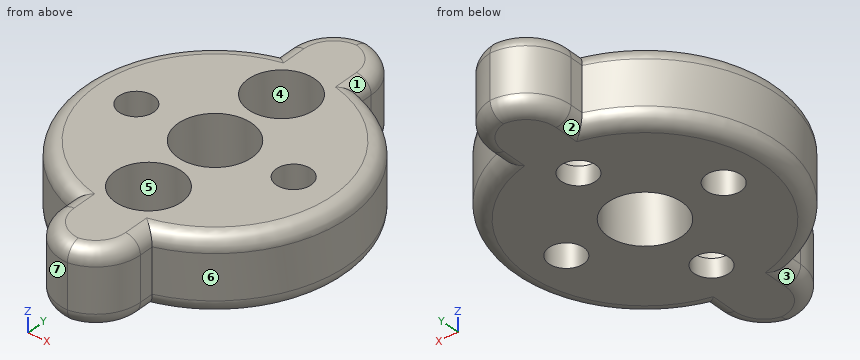
Autodesk Inventor part; units mm, degrees
ref_plane "YZ Plane" through (0, 0, 0) normal (1, 0, 0) x (0, 1, 0)
ref_plane "XZ Plane" through (0, 0, 0) normal (0, 1, 0) x (-1, 0, 0)
ref_plane "XY Plane" through (0, 0, 0) normal (0, 0, 1) x (1, 0, 0)
sketch "Sketch1" plane through (0, 0, 0) normal (0, 0, 1) x (1, 0, 0)
  circle A0 centre (0, 0) radius 11.43
  circle A1 centre (-6.75, 0) radius 1.5
  circle A2 centre (0, 0) radius 1.5
  circle A3 centre (6.75, 0) radius 1.5
  line L0 (0, 0) -> (0, 6.985)
  line L1 (0, 0) -> (0, -6.985)
  circle A4 centre (0, 6.985) radius 1.4986
  circle A5 centre (0, -6.985) radius 1.4986
  circle A6 centre (0, 0) radius 3.175
  arc A7 (0.31, -15.875) -> (3.5, -12.1158) centre (-0.31, -12.1158) ccw
  line L2 (3.5, -12.1158) -> (3.5, 12.1158)
  arc A8 (3.5, 12.1158) -> (0.31, 15.875) centre (-0.31, 12.1158) ccw
  arc A9 (0.31, 15.875) -> (-3.5, 12.065) centre (0.31, 12.065) ccw
  line L3 (-3.5, 12.065) -> (-3.5, -12.065)
  arc A10 (-3.5, -12.065) -> (0.31, -15.875) centre (0.31, -12.065) ccw
  circle A11 centre (0, 6.985) radius 1.5
  circle A12 centre (0, -6.985) radius 1.5
  line L4 (3.5, 0) -> (-3.5, 0)
  line L5 (0, 0) -> (0, 6.985)
  point P0 (3.5, -10.8809)
  point P1 (-3.5, -10.8809)
  point P2 (-3.5, 10.8809)
  point P3 (3.5, 10.8809)
  dimension "d0" = 22.86
  dimension "d1" = 6.985
  dimension "d2" = 6.985
  dimension "d3" = 2.9972
  dimension "d4" = 2.9972
  dimension "d7" = 6.35
extrude "Extrusion1" add sketch "Sketch1" along normal blind 6.35 contours A0 L2 | L2 L4 A6 L3 A0 | A0 L3 A9 A8 L2 | L2 A7 A10 L3 A0 | A0 L3 L4 A6 L2 | L3 A0
fillet "Fillet2" radius 1.27 20 edges at (11.43, 0, 0) (11.43, 0, 6.35) (-11.43, 0, 0) (-11.43, 0, 6.35) (3.5, 11.4984, 6.35) (2.595, 14.5809, 6.35) (-3.5, 11.473, 6.35) (-2.3841, 14.7591, 6.35) (-3.5, 11.473, 0) (-2.3841, 14.7591, 0) (3.5, 11.4984, 0) (2.595, 14.5809, 0) (2.595, -14.5809, 6.35) (3.5, -11.4984, 6.35) (-3.5, -11.473, 6.35) (-2.3841, -14.7591, 6.35) (3.5, -11.4984, 0) (2.595, -14.5809, 0) (-3.5, -11.473, 0) (-2.3841, -14.7591, 0)
sketch "Sketch3" plane through (0, 0, 6.35) normal (0, 0, 1) x (1, 0, 0)
  circle A0 centre (0, 6.985) radius 1.4986
  circle A1 centre (0, 6.985) radius 2.8575
  circle A2 centre (0, -6.985) radius 1.4986
  circle A3 centre (0, -6.985) radius 2.8575
  point P0 (0, 0)
  dimension "d12" = 5.715
  dimension "d13" = 5.715
extrude "Extrusion2" cut sketch "Sketch3" against normal blind 4.7625
properties part number "turning_cap"
The model under review builds one solid part; all positions refer to its coordinate system, in mm. Face numbers are marked on the shaded views. A direction names the side the tool comes from. Give positions to 0.01 mm unless a question says otherwise; leave off trailing zeros. Write each loop counter-clockwise with the first axis right and the second up, starting at its lowest first coordinate (ties: lowest second). Pieces come first, ordered by that corner, then holes. Notation, with made-up numbers: (-19.5, 32.25) -> (-0.5, 32.25) arc R23 ccw to (-0.5, 41.25) -> close; hole circle Ø8 at (73, 49.25). An arc over 180 degrees is marked (long way). Answer in a Markdown table with one row per item.
1) Mouldability with a two-part tool opening along Y and no side actions: class the marked faces 5, 6 and 7 as +Y half, -Y half, draft (parallel to the pull), parting line (faces both ways), or undercut.
Worked answers:
| item | result |
|---|---|
| face 5 | undercut |
| face 6 | parting line |
| face 7 | -Y half |
2) For L1, parallel to Y at x = -7.5, z = 5; L2, parallel to Z at x = 1.5, y = 14; L3, parallel to Y at x = 1, z = 6, list the stretches that pass through material, from the lowest coordinate up. Write a range as [from, to].
Worked answers:
| item | result |
|---|---|
| L1 | [-8.63, -1.3], [1.3, 8.63] |
| L2 | [0, 6.35] |
| L3 | [-15.27, -9.66], [-4.31, -3.01], [3.01, 4.31], [9.66, 15.27] |
3) Clearance check with flat-ended pins moving along their axes: P1, Ø3.5, axis at x = 0, y = -6.985, coming from the +Z side; P2, Ø4, axis at x = -5, y = -12, coming from the -Z side; P3, Ø0.9, axis at y = -11.5, z = 3, coming from the -X side; P4, Ø1.8, axis at x = 0, y = -6.985, coming from the -Z side. State where each tip first meets the part, or that it passes through.
Worked answers:
| item | result |
|---|---|
| P1 | z = 1.59 |
| P2 | z = 0.26 |
| P3 | x = -3.5 |
| P4 | through |
4) Tool access review of the marked faces 1, 2, 3 and 4: name each direction out of +Z, -Z, +X, -X, +Y, -Y from which nothing blocks a thin tool from reaching the whole face with its end or side.
Worked answers:
| item | result |
|---|---|
| face 1 | +Z, +X, +Y |
| face 2 | -Z, -X, +Y |
| face 3 | -Z, -X, -Y |
| face 4 | +Z |
5) Add section A-A on y = 0. State the section outline as (x, z) points (3 decimals), plus the area to 3 significant figures.
Worked answers:
| item | result |
|---|---|
| outline | (-11.43, 1.27) arc R1.27 ccw to (-10.16, 0) -> (-8.25, 0) -> (-8.25, 6.35) -> (-10.16, 6.35) arc R1.27 ccw to (-11.43, 5.08) -> close; (-5.25, 0) -> (-3.175, 0) -> (-3.175, 6.35) -> (-5.25, 6.35) -> close; (3.175, 0) -> (5.25, 0) -> (5.25, 6.35) -> (3.175, 6.35) -> close; (8.25, 0) -> (10.16, 0) arc R1.27 ccw to (11.43, 1.27) -> (11.43, 5.08) arc R1.27 ccw to (10.16, 6.35) -> (8.25, 6.35) -> close |
| area | 65.4 mm² |
6) Add section B-B on z = 4.75. Count the separate pieces of the cut face and the enclosed holes in it, plus the area to 3 significant figures.
Worked answers:
| item | result |
|---|---|
| separate pieces | 1 |
| enclosed holes | 5 |
| area | 366 mm² |
